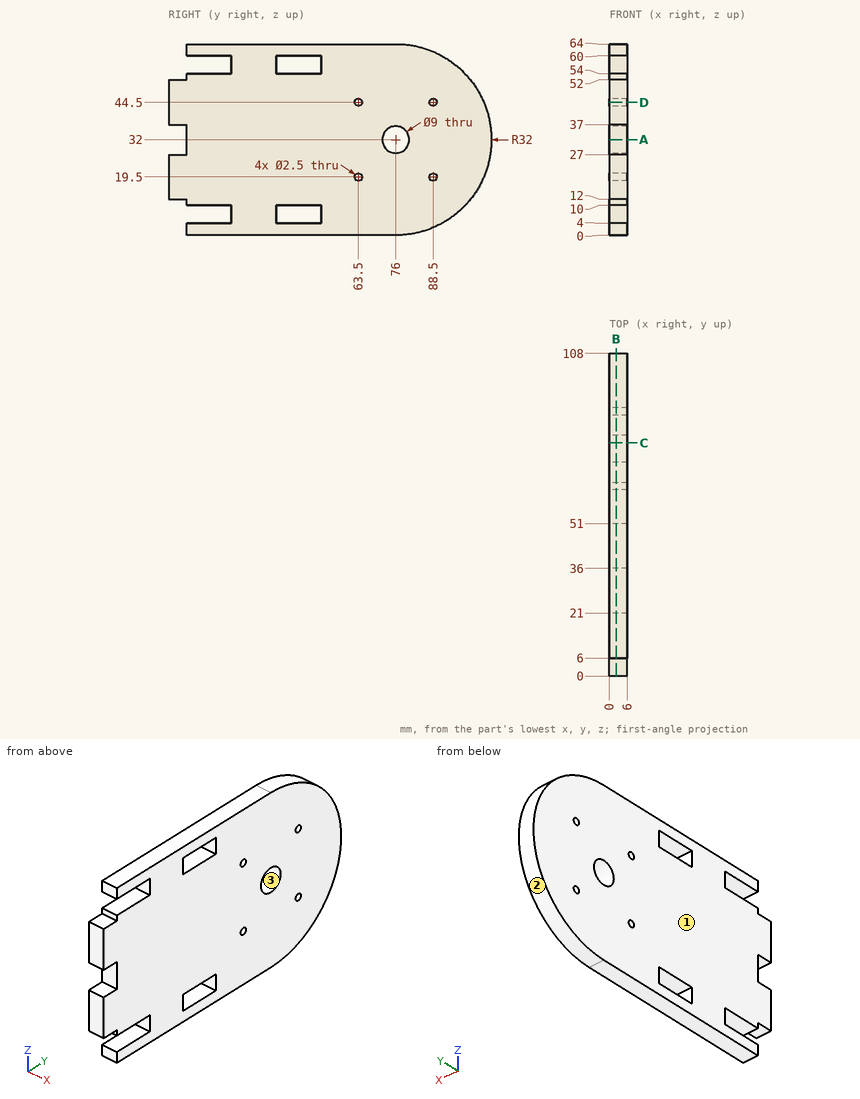
Check sheet for the drawn part. Datum: minimum x, y, z corner. Units: mm. Round coordinates to 2 decimals unless told otherwise and drop trailing zeros. Write each loop counter-clockwise with the first axis right and the second up, starting at its lowest first coordinate (ties: lowest second). Pieces come first, ordered by that corner, then holes. Notation, with made-up numbers: (-17.75, 81) -> (-7.75, 81) arc R34 cw to (-7.75, 113) -> close; hole circle Ø2 at (-3.5, 44). An arc over 180 degrees is marked (long way). Put each result on its own line as item: value.
(1) Go/stop test with flat-tipped pins: pin 1 Ø1.8 at (x, z) = (3.5, 33.5) entering from -Y; pin 2 Ø3 at (x, z) = (2, 7) entering from +Y; pin 3 Ø1 at (y, z) = (51, 55) entering from -X; pin 4 Ø2 at (x, y) = (4.5, 80) entering from -Z. Record where each tip stops, or that it passes through.
Values found:
pin 1: stops at y = 6
pin 2: stops at y = 97.72
pin 3: stops at x = 0
pin 4: stops at z = 0.14
(2) Material ranges on line 1 (Z direction, x = 3.5, y = 43); line 2 (Y direction, x = 3.6, z = 19.5); line 3 (Y direction, x = 1.4, z = 19), recorded low to high.
Values found:
line 1: z = 0 to 4, 10 to 54, 60 to 64
line 2: y = 0 to 62.25, 64.75 to 87.25, 89.75 to 105.46
line 3: y = 0 to 62.35, 64.65 to 87.35, 89.65 to 105.24
(3) Sectioned sample at B-B (x = 2.25). Count the separate pieces of the cut face and the enclosed holes in it, plus the area to 3 significant figures.
Values found:
separate pieces: 1
enclosed holes: 7
area: 5,830 mm^2
(4) Sectioned sample at C-C (y = 78). Enter the section's corners in (x, z).
Values found:
outline: (0, 0.06) -> (6, 0.06) -> (6, 27.97) -> (0, 27.97) -> close; (0, 36.03) -> (6, 36.03) -> (6, 63.94) -> (0, 63.94) -> close
(5) Mould release check, pull along Z, two halves, no side actions. Record for the marked faces 1, 2 and 3: released by +Z, released by -Z, zero draft, split by the parting line, or undercut.
Values found:
face 1: zero draft
face 2: split by the parting line
face 3: undercut
(6) Sectioned sample at D-D (z = 44.5). Enter the section's corners in (x, y), plus the area to 3 significant figures.
Values found:
outline: (0, 0) -> (6, 0) -> (6, 62.25) -> (0, 62.25) -> close; (0, 64.75) -> (6, 64.75) -> (6, 87.25) -> (0, 87.25) -> close; (0, 89.75) -> (6, 89.75) -> (6, 105.46) -> (0, 105.46) -> close
area: 603 mm^2
(7) Sectioned sample at A-A (z = 32). Enter the section's corners in (x, y).
Values found:
outline: (0, 6) -> (6, 6) -> (6, 71.5) -> (0, 71.5) -> close; (0, 80.5) -> (6, 80.5) -> (6, 108) -> (0, 108) -> close
